Autodesk Inventor part; units mm, degrees
ref_plane "Arbeitsebene1" through (0, 0, -3.5) normal (0, 0, -1) x (-1, 0, 0)
ref_plane "YZ Plane" through (0, 0, 0) normal (1, 0, 0) x (0, 1, 0)
ref_plane "XZ Plane" through (0, 0, 0) normal (0, 1, 0) x (-1, 0, 0)
sketch "Skizze4" plane through (0, 0, 0) normal (0, 1, 0) x (-1, 0, 0)
  line L0 (0, 0) -> (8, 0)
  line L1 (8, 0) -> (8, 7)
  line L2 (0, 0) -> (0, 7)
  line L3 (6.5, 10) -> (1.5, 10)
  line L4 (0, 7) -> (1.5, 10)
  line L5 (6.5, 10) -> (8, 7)
  dimension "d4" = 8
  dimension "d5" = 5
  dimension "d6" = 10
  dimension "d7" = 1.5
extrude "Extrusion2" add sketch "Skizze4" along normal blind 5.08
sketch "Skizze5" plane through (0, 0, 0) normal (0, -1, 0) x (1, 0, 0)
  line L0 (-7, 0) -> (-6, 0)
  line L1 (-6, 0) -> (-6, 7)
  line L2 (-6, 7) -> (-7, 7)
  line L3 (-7, 7) -> (-7, 0)
  line L4 (0, 0) -> (-8, 0)
  line L5 (-8, 0) -> (-8, 7)
  dimension "d10" = 7
  dimension "d11" = 1
  dimension "d12" = 1
extrude "Extrusion3" add sketch "Skizze5" along normal blind 0.5
sketch "Skizze6" plane through (0, 5.08, 0) normal (0, 1, 0) x (1, 0, 0)
  line L0 (-7, 0) -> (-7, -7)
  line L1 (-7, 0) -> (-6, 0)
  line L2 (-6, -7) -> (-6, 0)
  line L3 (-7, -7) -> (-6, -7)
  line L4 (-6, -7) -> (-7, -7)
  line L5 (-7, -7) -> (-7, 0)
  line L6 (-7, 0) -> (-6, 0)
  line L7 (-6, 0) -> (-6, -7)
  point P0 (0, 0)
extrude "Extrusion4" cut sketch "Skizze6" against normal blind 0.5
sketch "Skizze7" plane through (0, 0, 7) normal (1, 0, 0) x (0, 0, -1)
  line L0 (1, 0.54) -> (6, 0.54)
  line L1 (6, 0.54) -> (6, 4.54)
  line L2 (6, 4.54) -> (1, 4.54)
  line L3 (1, 4.54) -> (1, 0.54)
  line L4 (0, 0) -> (7, 0)
  line L5 (7, 0) -> (7, 5.08)
  dimension "d17" = 5
  dimension "d18" = 4
  dimension "d19" = 0.54
  dimension "d20" = 1
extrude "Extrusion5" cut sketch "Skizze7" against normal blind 1.5
sketch "Skizze8" plane through (-1.5, 0, 7) normal (1, 0, 0) x (0, 0, -1)
  circle A0 centre (4, 2.54) radius 1.5
  line L0 (1, 4.54) -> (6, 4.54)
  line L1 (6, 4.54) -> (6, 0.54)
  point P0 (7, 0)
  dimension "d23" = 3
  dimension "d24" = 2
  dimension "d25" = 2
extrude "Extrusion6" cut sketch "Skizze8" against normal blind 4
sketch "Skizze10" plane through (-5.5, 2.54, 3) normal (1, 0, 0) x (0, 0, -1)
  line L0 (-2.5, -1.5) -> (-0.5, -1.5)
  line L1 (-0.5, -1.5) -> (-0.5, 1.5)
  line L2 (-0.5, 1.5) -> (-2.5, 1.5)
  line L3 (-2.5, 1.5) -> (-2.5, -1.5)
  line L4 (2, 2) -> (2, -2)
  line L5 (-3, 2) -> (2, 2)
  point P0 (3, -2.54)
  dimension "d28" = 2
  dimension "d34" = 2.5
  dimension "d41" = 0.5
  dimension "d42" = 3
extrude "Extrusion7" add sketch "Skizze10" along normal blind 5
chamfer "Fase2" distance 0.5 angle 45 1 edges at (-0.5, 2.54, 3.5)
chamfer "Fase3" distance 1 angle 45 1 edges at (-0.5, 2.54, 5.5)
sketch "Skizze11" plane through (-6.5, 0, 10) normal (0, 0, 1) x (1, 0, 0)
  circle A0 centre (2.5, 2.54) radius 1.5
  line L0 (0, 5.08) -> (5, 5.08)
  line L1 (6.5, 0) -> (6.5, 5.08)
  line L2 (0, 0) -> (5, 0)
  dimension "d43" = 3
  dimension "d45" = 4
  dimension "d54" = 2.54
extrude "Extrusion8" cut sketch "Skizze11" against normal blind 1.5
sketch "Skizze12" plane through (-4, 2.54, 8.5) normal (0, 0, 1) x (1, 0, 0)
  line L0 (0.7826, 1.0062) -> (-0.3354, -1.2298)
  line L1 (-0.3354, -1.2298) -> (-0.7826, -1.0062)
  line L2 (-0.7826, -1.0062) -> (0.3354, 1.2298)
  line L3 (0.3354, 1.2298) -> (0.7826, 1.0062)
  line L4 (-0.3354, -1.2298) -> (0.3354, 1.2298) construction
  line L5 (-0.7826, -1.0062) -> (0.7826, 1.0062) construction
  line L6 (-2.5, 2.54) -> (2.5, 2.54)
  line L7 (4, -2.54) -> (4, 2.54)
  line L8 (-2.5, -2.54) -> (2.5, -2.54)
  point P0 (0, 0)
  point P1 (0, 0)
  point P2 (0, 0)
  dimension "d48" = 2.5
  dimension "d49" = 0.5
  dimension "d51" = 4
  dimension "d55" = 2.54
extrude "Extrusion9" cut sketch "Skizze12" against normal blind 0.5
sketch "Skizze14" plane through (0, 0, 0) normal (0, 0, -1) x (-1, 0, 0)
  line L0 (4.5, 2.04) -> (3.5, 2.04)
  line L1 (3.5, 2.04) -> (3.5, 3.04)
  line L2 (3.5, 3.04) -> (4.5, 3.04)
  line L3 (4.5, 3.04) -> (4.5, 2.04)
  line L4 (0, 0) -> (6, 0)
  line L5 (0, 0) -> (0, 5.08)
  dimension "d56" = 1
  dimension "d57" = 1
  dimension "d58" = 2.04
  dimension "d59" = 3.5
extrude "Extrusion10" add sketch "Skizze14" along normal blind 4
chamfer "Fase4" distance 0.25 angle 45 4 edges at (-3.5, 2.54, -4) (-4, 2.04, -4) (-4.5, 2.54, -4) (-4, 3.04, -4)
ref_plane "Arbeitsebene1" through (0, 0, -3.5) normal (0, 0, -1) x (-1, 0, 0)
sketch "Skizze15" plane through (0, 0, -3.5) normal (0, 0, -1) x (-1, 0, 0)
  circle A0 centre (4, 2.54) radius 0.55
  line L0 (3.5, 3.04) -> (3.5, 2.04)
  line L1 (3.5, 3.04) -> (4.5, 3.04)
  point P0 (0, 0)
  dimension "d66" = 1.1
  dimension "d67" = 0.5
  dimension "d68" = 0.5
extrude "Extrusion11" add sketch "Skizze15" against normal blind 0.5 contours A0 L0 L1 | L1 A0 | A0 L0 picked at (4.1108, 2.456)
properties part number "Schraubklemme_Blau_300V_16A"
Geometry check sheet. Reference: the model listing, model coordinates, mm. A direction names the side the tool comes from. Give positions to 0.01 mm unless a question says otherwise; leave off trailing zeros. Order: outer loops, then holes, each group sorted by start corner. A loop starts at its lowest first (then second) coordinate and runs counter-clockwise, first axis right, second up. Notation, with made-up numbers: M 39.5,-33 L 64.5,-33 A23 cw 64.5,-2 Z; hole C 37.5,-22 d7. An arc over 180 degrees is marked long. Use a Markdown table: item, result.
Item 1: Section check B-B (x = -5). Record the cut outline in (y, z).
Answers follow:
| item | result |
|---|---|
| outline | M 0,0 L 5.08,0 L 5.08,10 L 3.66,10 L 3.66,8.5 L 1.42,8.5 L 1.42,10 L 0,10 Z; hole M 1.13,3.5 A1.5 ccw long 3.95,3.5 Z |
Item 2: Material ranges on line 1 along Y through (x, z) = (-4, 9.7); line 2 along Z through (x, y) = (-0.5, 4.1); line 3 along X through (y, z) = (4.8, 0.75), recorded low to high.
Answers follow:
| item | result |
|---|---|
| line 1 | y = 0 to 1.04, 4.04 to 5.08 |
| line 2 | z = 0 to 1, 6 to 8 |
| line 3 | x = -8 to -7, -6 to 0 |
Item 3: Draft check along Y on faces 1 (the flat face through (-1, 4.04, 4)), 2 (the flat face through (-4, 5.08, 5)), 3 (the flat face through (-1, 3, 5)), 4 (the flat face through (-4, 2.04, -2)). Enter one of: +Y half, -Y half, draft (parallel to the pull), parting line (faces both ways), or undercut.
Answers follow:
| item | result |
|---|---|
| face 1 | undercut |
| face 2 | +Y half |
| face 3 | undercut |
| face 4 | -Y half |
Item 4: Section check C-C (y = 0.25). Record the cut outline in (x, z), and give its area (3 significant figures).
Answers follow:
| item | result |
|---|---|
| outline | M -8,0 L 0,0 L 0,7 L -1.5,10 L -6.5,10 L -8,7 Z |
| area | 75.5 mm2 |
Item 5: Section check A-A (z = 3). Record the cut outline in (x, y).
Answers follow:
| item | result |
|---|---|
| outline | M -8,0 L -7,0 L -7,-0.5 L -6,-0.5 L -6,0 L 0,0 L 0,0.54 L -1.5,0.54 L -1.5,1.04 L -5.5,1.04 L -5.5,4.04 L -1.5,4.04 L -1.5,4.54 L 0,4.54 L 0,5.08 L -6,5.08 L -6,4.58 L -7,4.58 L -7,5.08 L -8,5.08 Z |
Item 6: Depth check by flat-ended pin: P1, Ø0.6, axis at y = 2.5, z = 4.5, coming from the +X side; P2, Ø2.5, axis at x = -4, y = 2.54, coming from the +Z side; P3, Ø2, axis at x = -3, y = 4, coming from the -Z side; P4, Ø1.7, axis at x = -3, y = 2, coming from the -Z side. Enter the tip coordinate at first touch or a pass-through.
Answers follow:
| item | result |
|---|---|
| P1 | stops at x = -0.5 |
| P2 | stops at z = 8.5 |
| P3 | stops at z = 0 |
| P4 | stops at z = -4 |
Item 7: Section check D-D (x = -6.25). Record the cut outline in (y, z).
Answers follow:
| item | result |
|---|---|
| outline | M -0.5,0 L 4.58,0 L 4.58,7 L 5.08,7 L 5.08,10 L 0,10 L 0,7 L -0.5,7 Z |
Item 8: Tool access check on faces 5 (the flat face through (-6.5, 4.58, 3.5)), 6 (the cylindrical face through (-3.5, 2.5, 1.5)), 7 (the flat face through (-4, 2.5, 8)), 8 (the flat face through (-8, 3, 3)). Record the directions out of +Z, -Z, +X, -X, +Y, -Y that give a thin tool (end or side, any length) a straight path to the whole face; none if there is none.
Answers follow:
| item | result |
|---|---|
| face 5 | -Z, +Y |
| face 6 | +X |
| face 7 | +Z |
| face 8 | +Z, -Z, -X, +Y, -Y |
